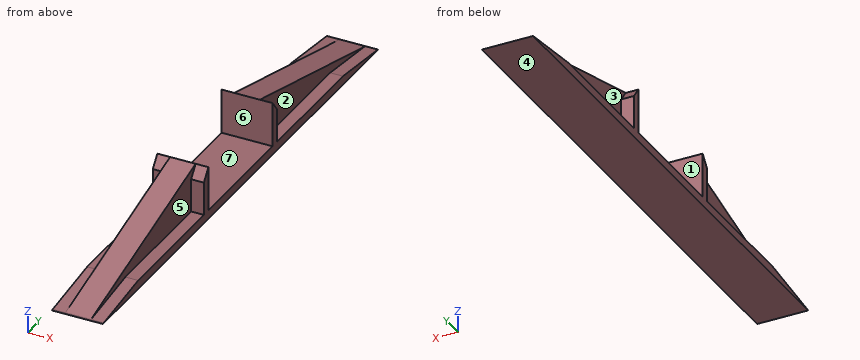
```python
from build123d import *

# Parameters (mm, degrees)
F0_W          = 30.9372
F0_H          = 2.1844
F1_DEPTH      = 6.35
F1_DEPTH_BACK = 6.35
F2_DEPTH      = 3.175
F2_DEPTH_BACK = 3.175


with BuildPart() as f1:
    # F0 (on Right) → F1 (new body, two sides)
    with BuildSketch(Plane.YZ) as f1_sk:
        Polygon((-50.8, 0), (0, 0), (0, 2.1844), (-2.1844, 2.1844), (-33.852487, 2.1844), (-50.437497, 0.095026), align=None)
        with Locations((15.4686, 1.0922)):
            Rectangle(F0_W, F0_H)
        Polygon((30.9372, 2.1844), (30.9372, 0), (81.7372, 0), (81.374697, 0.095026), (64.789687, 2.1844), (33.1216, 2.1844), align=None)
        Polygon((30.9372, 13.316668), (30.9372, 2.1844), (33.1216, 2.1844), (33.1216, 10.485845), align=None)
        Polygon((-2.1844, 2.1844), (0, 2.1844), (0, 13.316668), (-2.1844, 10.485845), align=None)
    extrude(amount=F1_DEPTH)
    extrude(f1_sk.sketch, amount=-F1_DEPTH_BACK)

    # F0 (on Right) → F2 (join, two sides)
    with BuildSketch(Plane.YZ) as f2_sk:
        Polygon((-2.1844, 10.485845), (0, 13.316668), (-50.437497, 0.095026), (-33.852487, 2.1844), (-10.214526, 8.380835), align=None)
        Polygon((81.374697, 0.095026), (30.9372, 13.316668), (33.1216, 10.485845), (41.151726, 8.380835), (64.789687, 2.1844), align=None)
        Polygon((33.1216, 10.485845), (33.1216, 2.1844), (64.789687, 2.1844), (41.151726, 8.380835), align=None)
        Polygon((-33.852487, 2.1844), (-2.1844, 2.1844), (-2.1844, 10.485845), (-10.214526, 8.380835), align=None)
    extrude(amount=F2_DEPTH)
    extrude(f2_sk.sketch, amount=-F2_DEPTH_BACK)


solid = f1.part
```
Verification items for the finished model (mm, model axes). Face numbers are marked on the shaded views. A direction names the side the tool comes from. Give positions to 0.01 mm unless a question says otherwise; leave off trailing zeros. Order: outer loops, then holes, each group sorted by start corner. A loop starts at its lowest first (then second) coordinate and runs counter-clockwise, first axis right, second up. Notation, with made-up numbers: M 65,27.5 L 69,27.5 A20 ccw 69,65.5 Z; hole C 56,81.5 d1. An arc over 180 degrees is marked long. Answer in a Markdown table with one row per item. Add a question column.
Item 1: Tool access check on the marked faces 1, 2, 3 and 4. Record the directions out of +Z, -Z, +X, -X, +Y, -Y that give a thin tool (end or side, any length) a straight path to the whole face; none if there is none.
Item 2: Section check A-A, the plane z = 7.5. Enter the section's corners in (x, y) (3 decimals), and give its area (3 significant figures).
Item 3: Mould release check, pull along Y, two halves, no side actions. Record for the marked faces 5, 6 and 7: released by +Y, released by -Y, zero draft, split by the parting line, or undercut.
Item 4: Section check C-C, the plane y = 70. Enter the section's corners in (x, z) (3 decimals), and give its area (3 significant figures).
Item 5: Section check D-D, the plane x = 5.25. Enter the section's corners in (y, z), and give its area (3 significant figures).
Item 6: Gauge pin test, flat ends, axial feed: pin 1 (3.5 mm diameter, centred on x = -4.5, y = 54.5, fed in from +Z); pin 2 (3.5 mm diameter, centred on x = 4.5, y = 48, fed in from +Z); pin 3 (1.5 mm diameter, centred on y = 40, z = 10.5, fed in from -X) (3 decimals); pin 4 (2 mm diameter, centred on y = 22, z = 5, fed in from +X). Record the tip position at first contact, or that the pin passes through.
Item 7: Section check B-B, the plane x = -0.75. Enter the section's corners in (y, z).
Item 8: Scan lines: probe 1 along Y at (x, z) = (4.5, 8); probe 2 along Z at (x, y) = (4.75, -23); probe 3 along X at (y, z) = (42, 4.5) (3 decimals). Record each from-to range of solid material in increasing order. Write a range as from..to.
Filled sheet:
| question | item | result |
|---|---|---|
| 1 | face 1 | +Z, +X, -X |
| 1 | face 2 | +Z, +X, +Y |
| 1 | face 3 | +Z, -X, +Y |
| 1 | face 4 | -Z, +X, -X, +Y, -Y |
| 2 | outline | M -6.35,-2.184 L -3.175,-2.184 L -3.175,-22.189 L 3.175,-22.189 L 3.175,-2.184 L 6.35,-2.184 L 6.35,0 L -6.35,0 Z; M -6.35,30.937 L 6.35,30.937 L 6.35,33.122 L 3.175,33.122 L 3.175,53.126 L -3.175,53.126 L -3.175,33.122 L -6.35,33.122 Z |
| 2 | area | 310 mm^2 |
| 3 | face 5 | zero draft |
| 3 | face 6 | undercut |
| 3 | face 7 | undercut |
| 4 | outline | M -6.35,0 L 6.35,0 L 6.35,1.528 L 3.175,1.528 L 3.175,3.077 L -3.175,3.077 L -3.175,1.528 L -6.35,1.528 Z |
| 4 | area | 29.2 mm^2 |
| 5 | outline | M -50.8,0 L 81.74,0 L 81.37,0.1 L 64.79,2.18 L 33.12,2.18 L 33.12,10.49 L 30.94,13.32 L 30.94,2.18 L 0,2.18 L 0,13.32 L -2.18,10.49 L -2.18,2.18 L -33.85,2.18 L -50.44,0.1 Z |
| 5 | area | 296 mm^2 |
| 6 | pin 1 | stops at z = 7.44 |
| 6 | pin 2 | stops at z = 9.14 |
| 6 | pin 3 | stops at x = -3.175 |
| 6 | pin 4 | passes through |
| 7 | outline | M -50.8,0 L 81.74,0 L 81.37,0.1 L 30.94,13.32 L 30.94,2.18 L 0,2.18 L 0,13.32 L -50.44,0.1 Z |
| 8 | probe 1 | y = -2.18..0, 30.94..33.12 |
| 8 | probe 2 | z = 0..2.18 |
| 8 | probe 3 | x = -3.175..3.175 |
